from build123d import *

# Parameters (mm, degrees)
F0_R     = 6.35
F1_DEPTH = 12.7


with BuildPart() as f1:
    # F0 (on Right) → F1 (new body)
    with BuildSketch(Plane.YZ):
        with BuildLine():
            ThreePointArc((-25.4, 0), (-4.965342, -24.909945), (23.458691, -9.739087))
            Line((23.458691, -9.739087), (38.047, 25.4))
            Line((38.047, 25.4), (38.047, 38.1))
            Line((38.047, 38.1), (23.458691, 73.239087))
            ThreePointArc((23.458691, 73.239087), (-4.965342, 88.409945), (-25.4, 63.5))
            Line((-25.4, 63.5), (-25.4, 0))
        make_face()
        Circle(F0_R, mode=Mode.SUBTRACT)
    extrude(amount=F1_DEPTH)


solid = f1.part
Source: CAD feature listing. Evaluate the final solid. Frame: model axes, mm. Round coordinates to 2 decimals unless told otherwise and drop trailing zeros. Loops run counter-clockwise (first coordinate to the right, second up) from the corner with the lowest first, then second, coordinate; pieces in that order, holes last. Notation, with made-up numbers: M -39,1 L -6,1 A17 cw -6,14 Z; hole C 14,68.5 d3. An arc over 180 degrees is marked long. Answer as CSV lines item,"result".
Q1. Contact query for flat-ended pins moving along their axis: pin 1 (3 mm diameter, centred on y = 12.5, z = 20.5, fed in from -X); pin 2 (4 mm diameter, centred on x = 5, z = 45.5, fed in from +Y). Output: stop coordinate, or through.
Verdict:
pin 1,"stops at x = 0"
pin 2,"stops at y = 35.81"
Q2. Cut plane C-C (z = 3). Return the cut outline in (x, y), plus the area to 3 significant figures.
Verdict:
outline,"M 0,-25.4 L 12.7,-25.4 L 12.7,-5.6 L 0,-5.6 Z; M 0,5.6 L 12.7,5.6 L 12.7,28.75 L 0,28.75 Z"
area,"546 mm^2"
Q3. Line query: line 1 along Z through (x, y) = (3, 0); line 2 along Y through (x, z) = (10.75, -0.5); line 3 along Y through (x, z) = (4.5, -2). Output: solid intervals per line, ascending.
Verdict:
line 1,"z = -25.4 to -6.35, 6.35 to 88.9"
line 2,"y = -25.4 to -6.33, 6.33 to 27.29"
line 3,"y = -25.32 to -6.03, 6.03 to 26.67"
Q4. Pull-direction query (Y, two-part tool) for faces 1 (the face through (6, -25.4, 32)), 2 (the face through (6.26, -5.44, -24.81)), 3 (the face through (6.26, -1.38, -6.2)); classes: +Y half, -Y half, draft (parallel to the pull), parting line (faces both ways), or undercut.
Verdict:
face 1,"-Y half"
face 2,"parting line"
face 3,"undercut"
Q5. Cut plane B-B (x = 3.5). Return the cut outline in (y, z), plus the area to 3 significant figures.
Verdict:
outline,"M -25.4,0 A25.4 ccw 23.46,-9.74 L 38.05,25.4 L 38.05,38.1 L 23.46,73.24 A25.4 ccw -25.4,63.5 Z; hole C 0,0 d12.7"
area,"5,680 mm^2"
Q6. Cut plane A-A (y = 0). Return the cut outline in (x, z), plus the area to 3 significant figures.
Verdict:
outline,"M 0,-25.4 L 12.7,-25.4 L 12.7,-6.35 L 0,-6.35 Z; M 0,6.35 L 12.7,6.35 L 12.7,88.9 L 0,88.9 Z"
area,"1,290 mm^2"
Q7. Cut plane D-D (z = 71). Return the cut outline in (x, y), plus the area to 3 significant figures.
Verdict:
outline,"M 0,-24.27 L 12.7,-24.27 L 12.7,24.39 L 0,24.39 Z"
area,"618 mm^2"
